CAD build for the part. Positions are in the model's coordinates, mm. Face numbers are marked on the shaded views. A direction names the side the tool comes from. Give positions to 0.01 mm unless a question says otherwise; leave off trailing zeros. Order: outer loops, then holes, each group sorted by start corner. A loop starts at its lowest first (then second) coordinate and runs counter-clockwise, first axis right, second up.
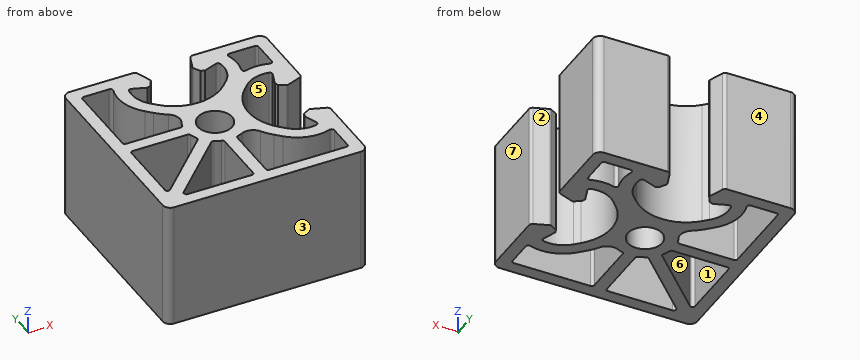
from build123d import *

# Parameters (mm, degrees)
SK_MAIN_EXTRUSION_R  = 3.4
MAIN_EXTRUSION_DEPTH = 25


with BuildPart() as part:
    # Sk Main Extrusion → Main Extrusion (new body)
    with BuildSketch(Plane.XY):
        with BuildLine():
            Line((16.671180212, 4.190076845), (19.506515107, 5.222054351))
            ThreePointArc((19.506515107, 5.222054351), (19.864364033, 5.496641489), (20, 5.926823816))
            Line((20, 5.926823816), (20, 18.5))
            ThreePointArc((20, 18.5), (19.560660172, 19.560660172), (18.5, 20))
            Line((18.5, 20), (5.926823816, 20))
            ThreePointArc((5.926823816, 20), (5.496641489, 19.864364033), (5.222054351, 19.506515107))
            Line((5.222054351, 19.506515107), (4.190076845, 16.671180212))
            ThreePointArc((4.190076845, 16.671180212), (4.175951325, 16.563886241), (4.208493649, 16.460675177))
            Line((4.208493649, 16.460675177), (4.987558066, 15.111296024))
            Line((4.987558066, 15.111296024), (5.718509166, 14.845251581))
            Line((5.718509166, 14.845251581), (8.396186179, 15.81984631))
            ThreePointArc((8.396186179, 15.81984631), (8.811074612, 15.786489799), (9.056960151, 15.450654467))
            ThreePointArc((9.056960151, 15.450654467), (8.933433013, 12.665882372), (7.504160339, 10.272684887))
            Line((7.504160339, 10.272684887), (6.540737726, 9.309262274))
            ThreePointArc((6.540737726, 9.309262274), (0, 6.6), (-6.540737726, 9.309262274))
            Line((-6.540737726, 9.309262274), (-7.504160339, 10.272684887))
            ThreePointArc((-7.504160339, 10.272684887), (-8.933433013, 12.665882372), (-9.056960151, 15.450654467))
            ThreePointArc((-9.056960151, 15.450654467), (-8.811074612, 15.786489799), (-8.396186179, 15.81984631))
            Line((-8.396186179, 15.81984631), (-5.718509166, 14.845251581))
            Line((-5.718509166, 14.845251581), (-4.987558066, 15.111296024))
            Line((-4.987558066, 15.111296024), (-4.208493649, 16.460675177))
            ThreePointArc((-4.208493649, 16.460675177), (-4.175951325, 16.563886241), (-4.190076845, 16.671180212))
            Line((-4.190076845, 16.671180212), (-5.222054351, 19.506515107))
            ThreePointArc((-5.222054351, 19.506515107), (-5.496641489, 19.864364033), (-5.926823816, 20))
            Line((-5.926823816, 20), (-18.5, 20))
            ThreePointArc((-18.5, 20), (-19.560660172, 19.560660172), (-20, 18.5))
            Line((-20, 18.5), (-20, -18.5))
            ThreePointArc((-20, -18.5), (-19.560660172, -19.560660172), (-18.5, -20))
            Line((-18.5, -20), (18.5, -20))
            ThreePointArc((18.5, -20), (19.560660172, -19.560660172), (20, -18.5))
            Line((20, -18.5), (20, -5.926823816))
            ThreePointArc((20, -5.926823816), (19.864364033, -5.496641489), (19.506515107, -5.222054351))
            Line((19.506515107, -5.222054351), (16.671180212, -4.190076845))
            ThreePointArc((16.671180212, -4.190076845), (16.563886241, -4.175951325), (16.460675177, -4.208493649))
            Line((16.460675177, -4.208493649), (15.111296024, -4.987558066))
            Line((15.111296024, -4.987558066), (14.845251581, -5.718509166))
            Line((14.845251581, -5.718509166), (15.81984631, -8.396186179))
            ThreePointArc((15.81984631, -8.396186179), (15.786489799, -8.811074612), (15.450654467, -9.056960151))
            ThreePointArc((15.450654467, -9.056960151), (12.665882372, -8.933433013), (10.272684887, -7.504160339))
            Line((10.272684887, -7.504160339), (9.309262274, -6.540737726))
            ThreePointArc((9.309262274, -6.540737726), (6.6, 0), (9.309262274, 6.540737726))
            Line((9.309262274, 6.540737726), (10.272684887, 7.504160339))
            ThreePointArc((10.272684887, 7.504160339), (12.665882372, 8.933433013), (15.450654467, 9.056960151))
            ThreePointArc((15.450654467, 9.056960151), (15.786489799, 8.811074612), (15.81984631, 8.396186179))
            Line((15.81984631, 8.396186179), (14.845251581, 5.718509166))
            Line((14.845251581, 5.718509166), (15.111296024, 4.987558066))
            Line((15.111296024, 4.987558066), (16.460675177, 4.208493649))
            ThreePointArc((16.460675177, 4.208493649), (16.563886241, 4.175951325), (16.671180212, 4.190076845))
        make_face()
        Circle(SK_MAIN_EXTRUSION_R, mode=Mode.SUBTRACT)
        with BuildLine():
            Line((-8.308504679, 7.441495321), (-9.444282589, 8.577273231))
            ThreePointArc((-9.444282589, 8.577273231), (-11.611987193, 12.430514315), (-11.464011904, 16.849169473))
            ThreePointArc((-11.464011904, 16.849169473), (-11.537349181, 17.295452819), (-11.940719521, 17.5))
            Line((-11.940719521, 17.5), (-17, 17.5))
            ThreePointArc((-17, 17.5), (-17.353553391, 17.353553391), (-17.5, 17))
            Line((-17.5, 17), (-17.5, 1.75))
            ThreePointArc((-17.5, 1.75), (-17.353553391, 1.396446609), (-17, 1.25))
            Line((-17, 1.25), (-6.156094541, 1.25))
            ThreePointArc((-6.156094541, 1.25), (-5.854730455, 1.351026708), (-5.675149655, 1.61328125))
            ThreePointArc((-5.675149655, 1.61328125), (-5.51245547, 2.10305366), (-5.307583096, 2.576734694))
            ThreePointArc((-5.307583096, 2.576734694), (-5.153883821, 4.359333373), (-6.230846881, 5.788120301))
            ThreePointArc((-6.230846881, 5.788120301), (-7.316529108, 6.555931161), (-8.308504679, 7.441495321))
        make_face(mode=Mode.SUBTRACT)
        with BuildLine():
            Line((17.5, 11.940719521), (17.5, 17))
            ThreePointArc((17.5, 17), (17.353553391, 17.353553391), (17, 17.5))
            Line((17, 17.5), (11.940719521, 17.5))
            ThreePointArc((11.940719521, 17.5), (11.537349181, 17.295452819), (11.464011904, 16.849169473))
            ThreePointArc((11.464011904, 16.849169473), (11.844928721, 14.508523804), (11.540116235, 12.156756572))
            ThreePointArc((11.540116235, 12.156756572), (11.66791097, 11.66791097), (12.156756572, 11.540116235))
            ThreePointArc((12.156756572, 11.540116235), (14.508523804, 11.844928721), (16.849169473, 11.464011904))
            ThreePointArc((16.849169473, 11.464011904), (17.295452819, 11.537349181), (17.5, 11.940719521))
        make_face(mode=Mode.SUBTRACT)
        with BuildLine():
            Line((-17.5, -1.75), (-17.5, -14.525126266))
            ThreePointArc((-17.5, -14.525126266), (-17.191341716, -14.987066032), (-16.646446609, -14.878679656))
            Line((-16.646446609, -14.878679656), (-5.236899672, -3.469132719))
            ThreePointArc((-5.236899672, -3.469132719), (-5.095239754, -3.18459946), (-5.153698917, -2.872174694))
            ThreePointArc((-5.153698917, -2.872174694), (-5.450889242, -2.257832251), (-5.675149655, -1.61328125))
            ThreePointArc((-5.675149655, -1.61328125), (-5.854730455, -1.351026708), (-6.156094541, -1.25))
            Line((-6.156094541, -1.25), (-17, -1.25))
            ThreePointArc((-17, -1.25), (-17.353553391, -1.396446609), (-17.5, -1.75))
        make_face(mode=Mode.SUBTRACT)
        with BuildLine():
            Line((-14.525126266, -17.5), (-1.75, -17.5))
            ThreePointArc((-1.75, -17.5), (-1.396446609, -17.353553391), (-1.25, -17))
            Line((-1.25, -17), (-1.25, -6.156094541))
            ThreePointArc((-1.25, -6.156094541), (-1.351026708, -5.854730455), (-1.61328125, -5.675149655))
            ThreePointArc((-1.61328125, -5.675149655), (-2.257832251, -5.450889242), (-2.872174694, -5.153698917))
            ThreePointArc((-2.872174694, -5.153698917), (-3.18459946, -5.095239754), (-3.469132719, -5.236899672))
            Line((-3.469132719, -5.236899672), (-14.878679656, -16.646446609))
            ThreePointArc((-14.878679656, -16.646446609), (-14.987066032, -17.191341716), (-14.525126266, -17.5))
        make_face(mode=Mode.SUBTRACT)
        with BuildLine():
            Line((1.75, -17.5), (17, -17.5))
            ThreePointArc((17, -17.5), (17.353553391, -17.353553391), (17.5, -17))
            Line((17.5, -17), (17.5, -11.940719521))
            ThreePointArc((17.5, -11.940719521), (17.295452819, -11.537349181), (16.849169473, -11.464011904))
            ThreePointArc((16.849169473, -11.464011904), (12.430514315, -11.611987193), (8.577273231, -9.444282589))
            Line((8.577273231, -9.444282589), (7.441495321, -8.308504679))
            ThreePointArc((7.441495321, -8.308504679), (6.555931161, -7.316529108), (5.788120301, -6.230846881))
            ThreePointArc((5.788120301, -6.230846881), (4.359333373, -5.153883821), (2.576734694, -5.307583096))
            ThreePointArc((2.576734694, -5.307583096), (2.10305366, -5.51245547), (1.61328125, -5.675149655))
            ThreePointArc((1.61328125, -5.675149655), (1.351026708, -5.854730455), (1.25, -6.156094541))
            Line((1.25, -6.156094541), (1.25, -17))
            ThreePointArc((1.25, -17), (1.396446609, -17.353553391), (1.75, -17.5))
        make_face(mode=Mode.SUBTRACT)
    extrude(amount=-MAIN_EXTRUSION_DEPTH)


solid = part.part
1. Saw through at C-C on x = 14. Give the cut face in (y, z), plus the area to 3 significant figures.
2. Mould opens along Y. For the marked faces 4, 5, 6 and 7 say: released by +Y, released by -Y, zero draft, split by the parting line, or undercut.
3. Saw through at D-D on y = 13. Give the cut face in (x, z), plus the area to 3 significant figures.
4. 3-axis set-ups, long thin cutter, end or side, ignore diameter. For the marked faces 1, 2 and 3: which of +Z, -Z, +X, -X, +Y, -Y reach the whole face in a straight line?
5. Pin check, flat tips, straight feed: P1, Ø5, axis at x = -2.5, y = 13.5, coming from the -Z side; P2, Ø5, axis at x = 9, y = -10, coming from the -Z side. Stop position of each tip, or through.
6. Saw through at A-A on x = 0. Give the cut face in (y, z), plus the area to 3 significant figures.
7. Wall check: line 1 (Y direction, x = 0, z = -6.5); line 2 (X direction, y = -17, z = -9.25); line 3 (X direction, y = -8, z = -22). Give the ranges that are in metal, low to high.
Reported:
1. outline: (-20, -25) - (-17.5, -25) - (-17.5, 0) - (-20, 0) - close; (-11.84, -25) - (-9.17, -25) - (-9.17, 0) - (-11.84, 0) - close; (9.17, -25) - (11.84, -25) - (11.84, 0) - (9.17, 0) - close; (17.5, -25) - (20, -25) - (20, 0) - (17.5, 0) - close
1. area: 259 mm2
2. face 4: released by +Y
2. face 5: undercut
2. face 6: undercut
2. face 7: zero draft
3. outline: (-20, -25) - (-17.5, -25) - (-17.5, 0) - (-20, 0) - close; (-11.73, -25) - (-9.02, -25) - (-9.02, 0) - (-11.73, 0) - close; (9.02, -25) - (11.73, -25) - (11.73, 0) - (9.02, 0) - close; (17.5, -25) - (20, -25) - (20, 0) - (17.5, 0) - close
3. area: 260 mm2
4. face 1: +Z, -Z
4. face 2: +Z, -Z, +X
4. face 3: +Z, -Z, +X, -X, -Y
5. P1: passes through
5. P2: stops at z = -25
6. outline: (-20, -25) - (-3.4, -25) - (-3.4, 0) - (-20, 0) - close; (3.4, -25) - (6.6, -25) - (6.6, 0) - (3.4, 0) - close
6. area: 495 mm2
7. line 1: y = -20 to -3.4, 3.4 to 6.6
7. line 2: x = -20 to -15.03, -1.25 to 1.25, 17.5 to 20
7. line 3: x = -20 to -17.5, -9.77 to -6.23, -1.25 to 1.25, 7.14 to 10.84, 15.68 to 20
